The listing builds one solid part. Answer for the finished solid, in the listing's coordinates (mm). Face numbers are marked on the shaded views. A direction names the side the tool comes from. Coordinates: 2 decimals unless noted, no trailing zeros. Loops run counter-clockwise (first coordinate to the right, second up) from the corner with the lowest first, then second, coordinate; pieces in that order, holes last. Notation, with made-up numbers: M 40,50.25 L 78,50.25 A5 cw 78,59.25 Z; hole C -19,32 d10. An arc over 180 degrees is marked long. Return JSON: item names as keys, results as strings. Group by question number.
1. Section A-A (x = 17.5) is taken. Write down the section's boundary in (y, z) (3 decimals), then the cut area to 3 significant figures.
2. Straight lines are drawn through the part: L1, parallel to Y at x = -40, z = 36; L2, parallel to X at y = -39.5, z = 9; L3, parallel to Y at x = -2.5, z = 19 (3 decimals). For each, find the intervals that lie inside material, in ascending order. Write a range as from..to.
3. Given P1, Ø1, axis at y = -48, z = 16.5, coming from the +X side; P2, Ø1.5, axis at x = 7, z = 1, coming from the +Y side; P3, Ø3, axis at x = 34, z = 15.5, coming from the +Y side, each flat-ended and moving along its own axis, determine where each tip first touches the part or whether it passes through.
4. Which of the six approach directions +Z, -Z, +X, -X, +Y, -Y give full straight-line access (tool end or side, diameter ignored) to the marked faces 1, 2 and 3?
5. Section B-B (y = -2) is taken. Count the separate pieces of the cut face and the enclosed holes in it, then the cut area to 3 significant figures.
6. The mould has two halves that part along Y. Classify the marked faces 4, 5 and 6: pulls with the +Y half, pulls with the -Y half, needs draft (parallel to the pull), parting line crosses it, or undercut.
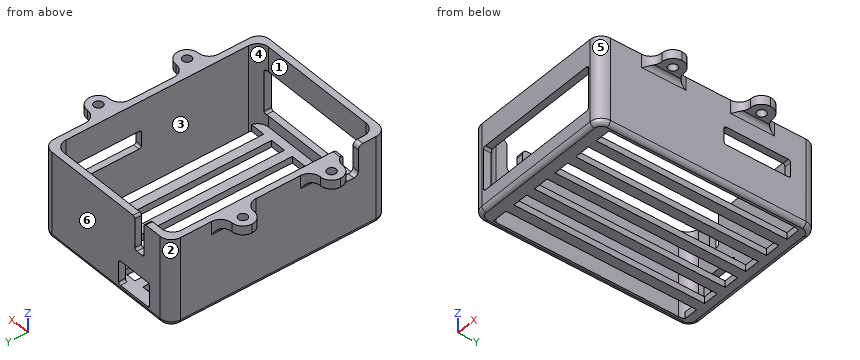
```python
from build123d import *

# Parameters (mm, degrees)
SKETCH1_W           = 7
SKETCH1_H           = 86
BOSS_EXTRUDE1_DEPTH = 3
SKETCH1_3_W         = 70
SKETCH1_3_H         = 98.29
SKETCH1_3_W_2       = 64
SKETCH1_3_H_2       = 92.29
BOSS_EXTRUDE2_DEPTH = 39.2
FILLET2_R           = 5
SKETCH2_W           = 58
SKETCH2_H           = 20
CUT_EXTRUDE1_DEPTH  = 64
FILLET3_R           = 1
SKETCH3_W           = 8
SKETCH3_H           = 30
CUT_EXTRUDE2_DEPTH  = 45
FILLET4_R           = 1
SKETCH4_W           = 5
SKETCH4_H           = 15
CUT_EXTRUDE3_DEPTH  = 81
FILLET5_R           = 1
SKETCH5_W           = 10
SKETCH5_H           = 10
SKETCH5_R           = 2
BOSS_EXTRUDE3_DEPTH = 4
FILLET6_R           = 5
FILLET7_R           = 5
FILLET8_R           = 2
FILLET9_R           = 2
SKETCH6_W           = 13.6
SKETCH6_H           = 7
CUT_EXTRUDE4_DEPTH  = 48
FILLET11_R          = 2
SKETCH7_W           = 17
SKETCH7_H           = 11
CUT_EXTRUDE5_DEPTH  = 60
FILLET12_R          = 1


with BuildPart() as part:
    # Sketch1 → Boss-Extrude1 (new body)
    with BuildSketch(Plane.XY):
        Polygon((-32, -46.145), (32, -46.145), (32, -42.355), (25, -42.355), (25, 43.645), (32, 43.645), (32, 46.145), (-32, 46.145), (-32, 43.645), (-25, 43.645), (-25, -42.355), (-32, -42.355), align=None)
        with Locations((-17.1, 0.645)):
            Rectangle(SKETCH1_W, SKETCH1_H, mode=Mode.SUBTRACT)
        with Locations((-5.7, 0.645)):
            Rectangle(SKETCH1_W, SKETCH1_H, mode=Mode.SUBTRACT)
        with Locations((5.7, 0.645)):
            Rectangle(SKETCH1_W, SKETCH1_H, mode=Mode.SUBTRACT)
        with Locations((17.1, 0.645)):
            Rectangle(SKETCH1_W, SKETCH1_H, mode=Mode.SUBTRACT)
    extrude(amount=BOSS_EXTRUDE1_DEPTH)

    # Sketch1<3> → Boss-Extrude2 (add)
    with BuildSketch(Plane.XY):
        Rectangle(SKETCH1_3_W, SKETCH1_3_H)
        Rectangle(SKETCH1_3_W_2, SKETCH1_3_H_2, mode=Mode.SUBTRACT)
    extrude(amount=BOSS_EXTRUDE2_DEPTH)

    # Fillet2
    fillet2_edges = [part.edges().sort_by_distance(p)[0] for p in [
        (-32, -46.145, 21.1),
        (32, -46.145, 21.1),
        (-32, 46.145, 21.1),
        (32, 46.145, 21.1),
        (35, -49.145, 19.6),
        (-35, -49.145, 19.6),
        (35, 49.145, 19.6),
        (-35, 49.145, 19.6),
    ]]
    fillet(fillet2_edges, radius=FILLET2_R)

    # Sketch2 → Cut-Extrude1 (cut)
    with BuildSketch(Plane(origin=(0, 0, 0), x_dir=(1, 0, 0), z_dir=(0, 1, 0))):
        with Locations((0, -18)):
            Rectangle(SKETCH2_W, SKETCH2_H)
    extrude(amount=-CUT_EXTRUDE1_DEPTH, mode=Mode.SUBTRACT)

    # Fillet3
    fillet3_edges = [part.edges().sort_by_distance(p)[0] for p in [
        (-29, -47.436287847, 28),
        (-29, -47.436287847, 8),
        (29, -47.436287847, 8),
        (29, -47.436287847, 28),
    ]]
    fillet(fillet3_edges, radius=FILLET3_R)

    # Sketch3 → Cut-Extrude2 (cut)
    with BuildSketch(Plane(origin=(0, 0, 0), x_dir=(0, 0, -1), z_dir=(1, 0, 0))):
        with Locations((-22, 22.145)):
            Rectangle(SKETCH3_W, SKETCH3_H)
    extrude(amount=CUT_EXTRUDE2_DEPTH, mode=Mode.SUBTRACT)

    # Fillet4
    fillet4_edges = [part.edges().sort_by_distance(p)[0] for p in [
        (33.5, 37.145, 26),
        (33.5, 7.145, 26),
        (33.5, 7.145, 18),
        (33.5, 37.145, 18),
    ]]
    fillet(fillet4_edges, radius=FILLET4_R)

    # Sketch4 → Cut-Extrude3 (cut)
    with BuildSketch(Plane(origin=(0, 0, 0), x_dir=(1, 0, 0), z_dir=(0, 1, 0))):
        with Locations((-18.5, -31.7)):
            Rectangle(SKETCH4_W, SKETCH4_H)
    extrude(amount=CUT_EXTRUDE3_DEPTH, mode=Mode.SUBTRACT)

    # Fillet5
    fillet5_edges = [part.edges().sort_by_distance(p)[0] for p in [
        (-16, 47.645, 39.2),
        (-21, 47.645, 39.2),
        (-16, 47.645, 24.2),
        (-21, 47.645, 24.2),
    ]]
    fillet(fillet5_edges, radius=FILLET5_R)

    # Sketch5 → Boss-Extrude3 (add)
    # profile 1 of 4: a face of its own
    with BuildSketch(Plane.XY.offset(39.2)):
        with Locations((40, 20)):
            Rectangle(SKETCH5_W, SKETCH5_H)
        with Locations((40, 20)):
            Circle(SKETCH5_R, mode=Mode.SUBTRACT)
    # profile 2 of 4: a face of its own
    with BuildSketch(Plane.XY.offset(39.2)):
        with Locations((40, -20)):
            Rectangle(SKETCH5_W, SKETCH5_H)
        with Locations((40, -20)):
            Circle(SKETCH5_R, mode=Mode.SUBTRACT)
    # profile 3 of 4: a face of its own
    with BuildSketch(Plane.XY.offset(39.2)):
        with Locations((-40, -20)):
            Rectangle(SKETCH5_W, SKETCH5_H)
        with Locations((-40, -20)):
            Circle(SKETCH5_R, mode=Mode.SUBTRACT)
    # profile 4 of 4: a face of its own
    with BuildSketch(Plane.XY.offset(39.2)):
        with Locations((-40, 20)):
            Rectangle(SKETCH5_W, SKETCH5_H)
        with Locations((-40, 20)):
            Circle(SKETCH5_R, mode=Mode.SUBTRACT)
    extrude(amount=-BOSS_EXTRUDE3_DEPTH)

    # Fillet6
    fillet6_edges = [part.edges().sort_by_distance(p)[0] for p in [
        (35, 15, 37.2),
        (35, 25, 37.2),
        (35, -25, 37.2),
        (35, -15, 37.2),
        (-35, -15, 37.2),
        (-35, -25, 37.2),
        (-35, 25, 37.2),
        (-35, 15, 37.2),
    ]]
    fillet(fillet6_edges, radius=FILLET6_R)

    # Fillet7
    fillet7_edges = [part.edges().sort_by_distance(p)[0] for p in [
        (-45, 25, 37.2),
        (-45, 15, 37.2),
        (-45, -15, 37.2),
        (-45, -25, 37.2),
        (45, -25, 37.2),
        (45, -15, 37.2),
        (45, 15, 37.2),
        (45, 25, 37.2),
    ]]
    fillet(fillet7_edges, radius=FILLET7_R - 0.0001)  # a hair under: the kernel refuses the full size

    # Fillet8
    fillet8_edges = [part.edges().sort_by_distance(p)[0] for p in [
        (35, 20, 35.2),
        (35, -20, 35.2),
        (-35, -20, 35.2),
        (-35, 20, 35.2),
    ]]
    fillet(fillet8_edges, radius=FILLET8_R)

    # Fillet9
    fillet9_edges = [part.edges().sort_by_distance(p)[0] for p in [
        (35, 0, 0),
        (-35, 0, 0),
        (0, 49.145, 0),
        (0, -49.145, 0),
        (-33.535533906, 47.680533906, 0),
        (33.535533906, 47.680533906, 0),
        (-33.535533906, -47.680533906, 0),
        (33.535533906, -47.680533906, 0),
    ]]
    fillet(fillet9_edges, radius=FILLET9_R)

    # Sketch6 → Cut-Extrude4 (cut)
    with BuildSketch(Plane(origin=(0, 0, 0), x_dir=(0, 0, -1), z_dir=(1, 0, 0))):
        with Locations((-32.4, -32.645)):
            Rectangle(SKETCH6_W, SKETCH6_H)
    extrude(amount=-CUT_EXTRUDE4_DEPTH, mode=Mode.SUBTRACT)

    # Fillet11
    fillet11_edges = [part.edges().sort_by_distance(p)[0] for p in [
        (-33.5, -29.145, 25.6),
        (-33.5, -36.145, 25.6),
        (-33.5, -36.145, 39.2),
        (-33.536822428, -29.145, 39.2),
    ]]
    fillet(fillet11_edges, radius=FILLET11_R)

    # Sketch7 → Cut-Extrude5 (cut)
    with BuildSketch(Plane(origin=(0, 0, 0), x_dir=(1, 0, 0), z_dir=(0, 1, 0))):
        with Locations((-15.5, -8.5)):
            Rectangle(SKETCH7_W, SKETCH7_H)
    extrude(amount=CUT_EXTRUDE5_DEPTH, mode=Mode.SUBTRACT)

    # Fillet12
    fillet12_edges = [part.edges().sort_by_distance(p)[0] for p in [
        (-24, 47.645, 14),
        (-7, 47.645, 3),
        (-24, 47.645, 3),
        (-7, 47.645, 14),
    ]]
    fillet(fillet12_edges, radius=FILLET12_R)


solid = part.part
```
Worked out:
{
 "1": {"outline": "M -49.145,2 A2 ccw -47.145,0 L -42.355,0 L -42.355,3 L -46.145,3 L -46.145,8 L -49.145,8 Z; M -49.145,28 L -46.145,28 L -46.145,39.2 L -49.145,39.2 Z; M 43.645,0 L 47.145,0 A2 ccw 49.145,2 L 49.145,39.2 L 46.145,39.2 L 46.145,3 L 43.645,3 Z", "area": "192 mm^2"},
 "2": {"L1": "-25..-22, -18..-15, 15..18, 22..25", "L2": "-35..-32, 32..35", "L3": "46.145..49.145"},
 "3": {"P1": "x = 33.71", "P2": "y = 49.13", "P3": "y = 48.48"},
 "4": {"face 1": "+Z", "face 2": "+Z, -Z, -X, +Y", "face 3": "+Z, -Z"},
 "5": {"separate pieces": "7", "enclosed holes": "0", "area": "299 mm^2"},
 "6": {"face 4": "undercut", "face 5": "pulls with the -Y half", "face 6": "pulls with the +Y half"}
}
